CAD build for the part. Positions are in the model's coordinates, mm. A direction names the side the tool comes from. Coordinates: 2 decimals unless noted, no trailing zeros. Loops run counter-clockwise (first coordinate to the right, second up) from the corner with the lowest first, then second, coordinate; pieces in that order, holes last. Notation, with made-up numbers: (-4.75, -25) -> (34.25, -25) arc R36 ccw to (34.25, 9) -> close; hole circle Ø8 at (47, 42). An arc over 180 degrees is marked (long way). Return JSON: item names as keys, results as strings. Group by question number.
(1) Tool access for faces 3 (the face through (-0.27, 5.99, 3.19)), 4 (the face through (-10.16, 29.11, 0.36)), 5 (the face through (-14, 19, 4.572)): list every direction of +Z, -Z, +X, -X, +Y, -Y with a clear straight run to the whole face (end or side of a thin tool).
(2) Saw through at B-B on z = 2.25. Give the number of separate pieces and of enclosed holes in the cut face, then the cut area to 3 significant figures.
(3) Saw through at A-A on y = 16.5. Write the cut outline in (x, z).
(4) Flat gauge pins, fed straight in: pin 1 Ø1.5 at (x, z) = (-7.5, 6.5) entering from +Y; pin 2 Ø2.5 at (x, y) = (-4.7, 28.69) entering from +Z; pin 3 Ø0.8 at (x, z) = (-15.5, 2.5) entering from -Y; pin 4 Ø0.8 at (x, z) = (-16, 3) entering from +Y. Where does each tip first touch, or does it go through?
(5) Saw through at D-D on y = 24.5. Write the cut outline in (x, z), then the cut area to 3 significant figures.
(6) Saw through at C-C on x = -3.5. Write the cut outline in (y, z), then the cut area to 3 significant figures.
(7) Mould opens along Y. For faces 1 (the face through (-15, 5, 8.433)), 2 (the face through (-2, 19, 4.572)) say: pulls with the +Y half, pulls with the -Y half, needs draft (parallel to the pull), parting line crosses it, or undercut.
(8) Probe L1, parallel to X at y = 30, z = 1.75; L2, parallel to Y at x = -14.75, z = 2.5; L3, parallel to X at y = 28.5, z = 4.25. List the from-to ranges inside material, lowest first.
Autodesk Inventor part; units mm, degrees
ref_plane "YZ Plane" through (0, 0, 0) normal (1, 0, 0) x (0, 1, 0)
ref_plane "XZ Plane" through (0, 0, 0) normal (0, 1, 0) x (-1, 0, 0)
ref_plane "XY Plane" through (0, 0, 0) normal (0, 0, 1) x (1, 0, 0)
sketch "Sketch1" plane through (0, 0, 0) normal (0, 0, 1) x (1, 0, 0)
  line L0 (-4.445, 2.3537) -> (-11.2171, 2.3537)
  line L1 (-16.0528, 3.6237) -> (-16.0528, 32.5162)
  line L2 (-11.2171, 33.8978) -> (-4.445, 33.8978)
  line L3 (0, 32.5162) -> (0, 3.6237)
  line L4 (-16.0528, 32.5162) -> (-11.2171, 33.8978)
  line L5 (-4.445, 33.8978) -> (0, 32.5162)
  line L6 (-16.0528, 3.6237) -> (-11.2171, 2.3537)
  line L7 (-4.445, 2.3537) -> (0, 3.6237)
  point P0 (0, 0)
  dimension "d13" = 28.8925
  dimension "d14" = 16.0528
  dimension "d15" = 28.8925
  dimension "d16" = 1.27
  dimension "d17" = 4.445
extrude "Extrusion1" add sketch "Sketch1" along normal blind 4.572
shell "Shell1" thickness 0.7112 removed faces 1 at (-8.9597, 23.3831, 4.572)
sketch "Sketch2" plane through (-11.1253, 3.0649, 0.7112) normal (0, 0, 1) x (1, 0, 0)
  circle A0 centre (3.0989, 7.3888) radius 0.762
  line L0 (-0.0918, -0.7112) -> (6.6803, -0.7112)
  line L1 (10.4141, 28.9276) -> (10.4141, 1.0953)
  line L2 (-4.2163, 1.1073) -> (-4.2163, 28.9148)
  circle A1 centre (3.0989, 16.2433) radius 0.9525
  line L3 (11.1253, 0.5588) -> (11.1253, 29.4513)
  line L4 (6.6803, -0.7112) -> (11.1253, 0.5588)
  line L5 (6.6803, 30.8329) -> (-0.0918, 30.8329)
  line L6 (-4.9275, 29.4513) -> (-4.9275, 0.5588)
  line L7 (3.0989, 30.8329) -> (3.0989, 0) construction
  line L8 (6.5806, 0) -> (0, 0)
  circle A2 centre (-3.2765, 20.0769) radius 0.762
  circle A3 centre (1.8543, 26.0069) radius 0.889
  circle A4 centre (6.4263, 25.6259) radius 0.762
  circle A5 centre (6.4263, 25.6259) radius 1.524
  arc A6 (0.4506, 27.0982) -> (1.8543, 27.7849) centre (1.8543, 26.0069) ccw
  arc A7 (-0.0507, 27.488) -> (1.8543, 28.4199) centre (1.8543, 26.0069) ccw
  line L9 (0.0078, 30.1217) -> (6.5723, 30.1217)
  line L10 (1.8543, 28.4199) -> (1.8543, 27.7849)
  line L11 (-0.0507, 27.488) -> (0.4506, 27.0982)
  line L12 (0.4506, 27.0982) -> (1.8456, 26.0137) construction
  arc A8 (-4.2163, 17.4457) -> (-4.2163, 22.7081) centre (-3.2765, 20.0769) ccw
  arc A9 (-4.2163, 18.1332) -> (-4.2163, 22.0206) centre (-3.2765, 20.0769) ccw
  point P0 (11.1253, -3.0649)
  point P1 (3.0989, 15.2908)
  point P2 (9.4743, 0.0871)
  dimension "d71" = 1.905
  dimension "d18" = 1.524
  dimension "d19" = 8.1
  dimension "d53" = 7.3152
  dimension "d54" = 14.6304
  dimension "d72" = 16.002
  dimension "d93" = 7.3152
  dimension "d98" = 3.556
  dimension "d99" = 0.635
  dimension "d100" = 4.572
  dimension "d101" = 0.381
  dimension "d102" = 3.9878
  dimension "d103" = 4.4958
  dimension "d104" = 1.905
  dimension "d105" = 2.032
  dimension "d106" = 0.635
sketch "Sketch3" plane through (-11.1253, 3.0649, 0.7112) normal (0, 0, 1) x (1, 0, 0)
  line L0 (6.5806, 0) -> (10.4141, 1.0953)
  line L1 (-4.2163, 1.1073) -> (0, 0)
  line L2 (10.4141, 28.9276) -> (10.4141, 1.0953)
  line L3 (-4.2163, 28.9148) -> (-4.2163, 1.1073)
  line L4 (6.5806, 0) -> (0, 0) construction
  circle A0 centre (9.7791, 15.2046) radius 0.635
  circle A1 centre (9.7791, 15.2046) radius 1.27
  circle A2 centre (-3.5813, 15.2046) radius 0.635
  circle A3 centre (-3.5813, 15.2046) radius 1.27
  line L5 (-4.2163, 1.1073) -> (-4.2163, 28.9148)
  circle A4 centre (-3.5813, 2.2053) radius 0.635
  circle A5 centre (-3.5813, 2.2053) radius 1.27
  circle A6 centre (9.7791, 2.2053) radius 0.635
  circle A7 centre (9.7791, 2.2053) radius 1.27
  circle A8 centre (-3.5813, 28.4359) radius 0.635
  circle A9 centre (-3.5813, 28.4359) radius 1.27
  circle A10 centre (9.7791, 28.46) radius 0.635
  circle A11 centre (9.7791, 28.46) radius 1.27
  line L6 (6.5723, 30.1217) -> (10.4141, 28.9276)
  line L7 (-4.2163, 28.9148) -> (0.0078, 30.1217)
  point P0 (11.1253, -3.0649)
  point P1 (10.4141, 16.3045)
  point P2 (10.4141, 14.1048)
  point P3 (10.4141, 15.2046)
  point P4 (-4.2163, 16.3045)
  point P5 (-4.2163, 15.2046)
  point P6 (-4.2163, 14.1048)
  point P7 (10.4141, 2.2053)
  point P8 (10.4141, 3.3052)
  point P9 (9.8642, 0.9382)
  point P10 (10.3762, 1.0844)
  point P11 (10.4141, 1.1055)
  point P12 (-3.5619, 0.9355)
  point P13 (-4.2163, 3.3052)
  point P14 (-4.2163, 2.2053)
  point P15 (9.9675, 29.0664)
  point P16 (8.9172, 29.3928)
  point P17 (10.4141, 27.3602)
  point P18 (10.4141, 28.46)
  point P19 (-2.6983, 29.3486)
  point P20 (-3.7558, 29.0464)
  point P21 (-4.2163, 28.4359)
  point P22 (-4.2163, 27.336)
  dimension "d57" = 1.27
  dimension "d58" = 0.635
  dimension "d59" = 1.27
  dimension "d60" = 0.635
  dimension "d63" = 1.27
  dimension "d64" = 0.635
  dimension "d65" = 1.27
  dimension "d66" = 0.635
  dimension "d67" = 1.27
  dimension "d68" = 0.635
  dimension "d69" = 1.27
  dimension "d70" = 0.635
extrude "Extrusion10" add sketch "Sketch3" along normal blind 7.7216 contours A6 | A0 | A10 | A4 | A2 | A8
extrude "Extrusion11" cut sketch "Sketch2" against normal up to surface (0.7112 mm away) contours A0 | A1 | A2 | A3 | A4
extrude "Extrusion12" add sketch "Sketch2" along normal blind 1.905 contours L2 A9 A8 | A5 | A6 L10 A7 L11
sketch "Sketch5" plane through (-16.0528, 3.6237, 0) normal (-1, 0, 0) x (0, 0, 1)
  line L0 (4.572, 14.6458) -> (4.572, 27.8771)
  line L1 (4.572, 23.5585) -> (3.302, 23.5585)
  line L2 (3.302, 13.3985) -> (4.572, 13.3985)
  line L3 (0, 28.8925) -> (4.572, 28.8925)
  line L4 (3.302, 22.4155) -> (0.7112, 22.4155)
  line L5 (1.778, 13.3985) -> (3.302, 13.3985)
  line L6 (1.778, 15.9385) -> (1.778, 13.3985)
  line L7 (4.572, 15.9385) -> (1.778, 15.9385)
  line L8 (0.7112, 17.0815) -> (4.572, 17.0815)
  line L9 (3.302, 23.5585) -> (3.302, 22.4155)
  line L10 (4.572, 13.3985) -> (4.572, 15.9385)
  line L11 (4.572, 17.0815) -> (4.572, 23.5585)
  line L12 (0.7112, 22.3121) -> (0.7112, 16.7241)
  line L13 (0.7112, 17.0815) -> (0.7112, 22.4155)
  point P0 (0, -3.6237)
  point P1 (0.7112, 22.1493)
  point P2 (0.7112, 16.8869)
  dimension "d109" = 5.334
  dimension "d114" = 1.143
extrude "Extrusion14" add sketch "Sketch3" along normal up to surface (3.8608 mm away) contours A6 | A7 L2 L0 | A11 L6 A10 L2 | L2 L6 A11 | A0 | A1 L2 | L0 A7 | A7 L2 | A10 L6 L2 | A10 | A4 | L3 A5 L1 | A5 L3 | A9 L7 L3 | L3 A8 L7 A9 | A3 L3 | A2 | L3 A3 | L1 A5 | L3 L7 A8 | A8 picked at (10.0816, 1.2114) picked at (10.1817, 14.2329)
extrude "Extrusion13" cut sketch "Sketch5" against normal up to surface (0.7112 mm away)
extrude "Extrusion15" cut sketch "Sketch5" along normal up to surface (0.7112 mm away) from surface at -16.0528
sketch "Sketch6" plane through (0, 0, 4.572) normal (0, 0, 1) x (1, 0, 0)
  line L0 (-0.7112, 6.37) -> (-0.7112, 17.1697)
  line L1 (0, 8.275) -> (-0.7112, 8.275)
  line L2 (-0.7112, 8.275) -> (-0.7112, 6.37)
  line L3 (0, 6.37) -> (0, 8.275)
  arc A0 (-0.7112, 6.37) -> (-1.261, 4.003) centre (-1.3462, 5.2702) ccw
  circle A1 centre (-14.7066, 5.2702) radius 0.635
  arc A2 (-0.7491, 4.1493) -> (-0.7112, 4.1703) centre (-1.3462, 5.2702) ccw
  line L4 (-0.7112, 4.1703) -> (-0.7112, 4.1601)
  line L5 (-0.7112, 4.1601) -> (-0.7491, 4.1493)
  circle A3 centre (-1.3462, 5.2702) radius 0.635
  line L6 (0, 17.0222) -> (-0.7112, 17.0222)
  line L7 (-0.7112, 17.0222) -> (-0.7112, 6.37)
  arc A4 (-0.7112, 6.37) -> (-1.261, 4.003) centre (-1.3462, 5.2702) ccw
  line L8 (-1.261, 4.003) -> (-4.5446, 3.0649)
  line L9 (-4.5446, 3.0649) -> (-11.1253, 3.0649)
  line L10 (-11.1253, 3.0649) -> (-14.6871, 4.0003)
  arc A5 (-14.6871, 4.0003) -> (-15.3416, 6.37) centre (-14.7066, 5.2702) ccw
  line L11 (-15.3416, 6.37) -> (-15.3416, 17.0222)
  line L12 (-15.3416, 17.0222) -> (-16.0528, 17.0222)
  line L13 (-16.0528, 17.0222) -> (-16.0528, 3.6237)
  line L14 (-16.0528, 3.6237) -> (-11.2171, 2.3537)
  line L15 (-11.2171, 2.3537) -> (-4.445, 2.3537)
  line L16 (-4.445, 2.3537) -> (0, 3.6237)
  line L17 (0, 3.6237) -> (0, 17.0222)
  arc A6 (-0.7112, 6.37) -> (-1.261, 4.003) centre (-1.3462, 5.2702) ccw construction
  circle A7 centre (-1.3462, 5.2702) radius 1.27 construction
  arc A8 (0, 5.4827) -> (-0.7112, 6.37) centre (-1.4943, 5.0137) ccw
  line L18 (0, 6.37) -> (0, 5.4827)
  line L19 (-8.0264, 33.8978) -> (-8.0264, 3.0649) construction
  line L20 (-16.0528, 8.275) -> (-15.3416, 8.275)
  line L21 (-16.0528, 6.37) -> (-16.0528, 8.275)
  line L22 (-15.3416, 8.275) -> (-15.3416, 6.37)
  line L23 (-16.0528, 5.4827) -> (-16.0528, 8.275)
  arc A9 (-15.3416, 6.37) -> (-16.0528, 5.4827) centre (-14.5585, 5.0137) ccw
  line L24 (-16.0528, 6.37) -> (-16.0528, 5.4827)
  point P0 (0, 0)
extrude "Extrusion16" cut sketch "Sketch6" against normal up to surface (2.794 mm away) contours L0 L1 L3 L17 A8 | A9 L13 L20 L11
properties part number "Back half gearbox"
Geometry results:
{
 "1": {"face 3": "+Z, +X", "face 4": "+Z, -Z", "face 5": "+Z"},
 "2": {"separate pieces": "10", "enclosed holes": "2", "area": "90.0 mm²"},
 "3": {"outline": "(-16.05, 0) -> (0, 0) -> (0, 4.57) -> (-0.71, 4.57) -> (-0.71, 0.71) -> (-15.34, 0.71) -> (-15.34, 4.57) -> (-16.05, 4.57) -> close"},
 "4": {"pin 1": "through", "pin 2": "z = 2.62", "pin 3": "y = 3.37", "pin 4": "y = 32.65"},
 "5": {"outline": "(-16.05, 0) -> (0, 0) -> (0, 0.71) -> (-11.96, 0.71) -> (-11.96, 2.62) -> (-12.72, 2.62) -> (-12.72, 0.71) -> (-16.05, 0.71) -> close", "area": "12.9 mm²"},
 "6": {"outline": "(2.62, 0) -> (33.6, 0) -> (33.6, 4.57) -> (32.86, 4.57) -> (32.86, 0.71) -> (29.63, 0.71) -> (29.63, 2.62) -> (27.75, 2.62) -> (27.75, 0.71) -> (3.36, 0.71) -> (3.36, 4.57) -> (2.62, 4.57) -> close", "area": "31.3 mm²"},
 "7": {"face 1": "needs draft", "face 2": "undercut"},
 "8": {"L1": "-16.05 to -15.34, -11.5 to -10.79, -7.75 to -7.04, -5.48 to -3.92, -0.71 to 0", "L2": "3.28 to 6.54, 17 to 19.54, 20.37 to 21.01, 25.27 to 25.91, 30.23 to 32.89", "L3": "-16.05 to -15.34, -0.71 to 0"}
}
